```python
from build123d import *

# Parameters (mm, degrees)
F0_W     = 13
F0_H     = 125.402425
F1_DEPTH = 6


with BuildPart() as f1:
    # F0 (on Front) → F1 (new body)
    with BuildSketch(Plane.XZ):
        Polygon((60.391705, 30.000078), (60.391705, 90.000078), (-9.955426, 90.000078), (-9.955426, -93.209804), (10.044574, -93.209804), (10.044574, 70.060078), (40.444729, 70.060078), (40.444729, 30.000078), align=None)
        with Locations((0.044574, -25.701134)):
            Rectangle(F0_W, F0_H, mode=Mode.SUBTRACT)
        Polygon((6.544574, 45.000078), (-6.455426, 45.000078), (-6.455426, 73.97807), (-6.455426, 86.500078), (56.891705, 86.500078), (56.891705, 73.97807), (56.891705, 45.000078), (43.944729, 45.000078), (43.944729, 73.560078), (6.544574, 73.560078), align=None, mode=Mode.SUBTRACT)
    extrude(amount=F1_DEPTH)


solid = f1.part
```
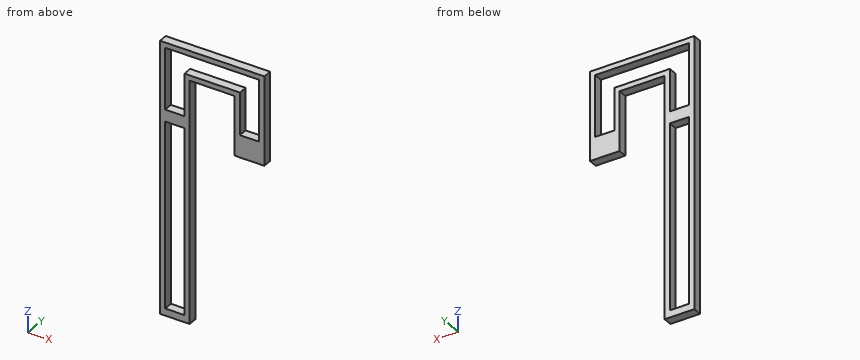
Could you check a few things on this model? Use its own coordinates, in mm. Give positions to 0.01 mm unless a question says otherwise; leave off trailing zeros. Order: outer loops, then holes, each group sorted by start corner. A loop starts at its lowest first (then second) coordinate and runs counter-clockwise, first axis right, second up.
Q1. Suppose I cut it at A-A, the plane x = 12. Write out the boundary of the cut face in (y, z).
Q2. Suppose I cut it at C-C, the plane x = 0.5. Write out the boundary of the cut face in (y, z), and give its area (3 significant figures).
Q3. Suppose I cut it at D-D, the plane y = -3.75. Write out the boundary of the cut face in (x, z), and give its area (3 significant figures).
Q4. Suppose I cut it at B-B, the plane z = -5. Write out the boundary of the cut face in (x, y), and give its area (3 significant figures).
Q5. I'm going to push flat-ended pins straight in: P1, Ø3, axis at x = 30, y = -4, coming from the -Z side; P2, Ø3, axis at x = 53, y = -3, coming from the -Z side. Where does each tip first touch, or does it pass through?
Q6. If I drill on line 1 along Z through (x, y) = (-6, -0.5); line 2 along Z through (x, y) = (15.5, -5.35); line 3 along X through (y, z) = (-0.65, 47.5), over which ranges is the centre line in solid material (lowest first)?
Solution:
1. outline: (-6, 70.06) - (0, 70.06) - (0, 73.56) - (-6, 73.56) - close; (-6, 86.5) - (0, 86.5) - (0, 90) - (-6, 90) - close
2. outline: (-6, -93.21) - (0, -93.21) - (0, -88.4) - (-6, -88.4) - close; (-6, 37) - (0, 37) - (0, 45) - (-6, 45) - close; (-6, 86.5) - (0, 86.5) - (0, 90) - (-6, 90) - close
2. area: 97.8 mm2
3. outline: (-9.96, -93.21) - (10.04, -93.21) - (10.04, 70.06) - (40.44, 70.06) - (40.44, 30) - (60.39, 30) - (60.39, 90) - (-9.96, 90) - close; hole (-6.46, -88.4) - (6.54, -88.4) - (6.54, 37) - (-6.46, 37) - close; hole (-6.46, 45) - (6.54, 45) - (6.54, 73.56) - (43.94, 73.56) - (43.94, 45) - (56.89, 45) - (56.89, 86.5) - (-6.46, 86.5) - close
3. area: 2,280 mm2
4. outline: (-9.96, -6) - (-6.46, -6) - (-6.46, 0) - (-9.96, 0) - close; (6.54, -6) - (10.04, -6) - (10.04, 0) - (6.54, 0) - close
4. area: 42.0 mm2
5. P1: stops at z = 70.06
5. P2: stops at z = 30
6. line 1: z = -93.21 to -88.4, 37 to 45, 86.5 to 90
6. line 2: z = 70.06 to 73.56, 86.5 to 90
6. line 3: x = -9.96 to -6.46, 6.54 to 10.04, 40.44 to 43.94, 56.89 to 60.39
